```python
from build123d import *

# Parameters (mm, degrees)
SKETCH1_W           = 360
SKETCH1_H           = 210
BOSS_EXTRUDE1_DEPTH = 1
SKETCH2_R           = 5
SKETCH2_R_2         = 2.3
BOSS_EXTRUDE2_DEPTH = 5.7


with BuildPart() as part:
    # Sketch1 → Boss-Extrude1 (new body)
    with BuildSketch(Plane(origin=(0, 0, 0), x_dir=(1, 0, 0), z_dir=(0, 1, 0))):
        Rectangle(SKETCH1_W, SKETCH1_H)
        Polygon((28, -45.5), (0, -45.5), (0, 45.5), (-78.4, 45.5), (-78.4, -7.9), (-95, -7.9), (-95, 79.1), (-78.4, 79.1), (-78.4, 68.1), (28, 68.1), (28, 45.5), (66.5, 45.5), (66.5, -45.5), (66.5, -97), (28, -97), align=None, mode=Mode.SUBTRACT)
    extrude(amount=BOSS_EXTRUDE1_DEPTH)

    # Sketch2 → Boss-Extrude2 (add)
    with BuildSketch(Plane(origin=(0, 1, 0), x_dir=(1, 0, 0), z_dir=(0, 1, 0))):
        with Locations((-71.4, 75.1)):
            Circle(SKETCH2_R)
        with Locations((-71.4, 75.1)):
            Circle(SKETCH2_R_2, mode=Mode.SUBTRACT)
        with Locations((-71.4, 38.5)):
            Circle(SKETCH2_R)
        with Locations((-71.4, 38.5)):
            Circle(SKETCH2_R_2, mode=Mode.SUBTRACT)
        with Locations((-102, 75.1)):
            Circle(SKETCH2_R)
        with Locations((-102, 75.1)):
            Circle(SKETCH2_R_2, mode=Mode.SUBTRACT)
        with Locations((-7, 38.5)):
            Circle(SKETCH2_R)
        with Locations((-7, 38.5)):
            Circle(SKETCH2_R_2, mode=Mode.SUBTRACT)
        with Locations((35, 52.5)):
            Circle(SKETCH2_R)
        with Locations((35, 52.5)):
            Circle(SKETCH2_R_2, mode=Mode.SUBTRACT)
        with Locations((21, -52.5)):
            Circle(SKETCH2_R)
        with Locations((21, -52.5)):
            Circle(SKETCH2_R_2, mode=Mode.SUBTRACT)
        with Locations((-71.4, -0.9)):
            Circle(SKETCH2_R)
        with Locations((-71.4, -0.9)):
            Circle(SKETCH2_R_2, mode=Mode.SUBTRACT)
        with Locations((-102, -0.9)):
            Circle(SKETCH2_R)
        with Locations((-102, -0.9)):
            Circle(SKETCH2_R_2, mode=Mode.SUBTRACT)
        with Locations((73.5, -90)):
            Circle(SKETCH2_R)
        with Locations((73.5, -90)):
            Circle(SKETCH2_R_2, mode=Mode.SUBTRACT)
        with Locations((21, -90)):
            Circle(SKETCH2_R)
        with Locations((21, -90)):
            Circle(SKETCH2_R_2, mode=Mode.SUBTRACT)
    extrude(amount=BOSS_EXTRUDE2_DEPTH)


solid = part.part
```
Design review of the part built by this model. Coordinates are the model's own, in mm. A direction names the side the tool comes from. Coordinates: 2 decimals unless noted, no trailing zeros. Order: outer loops, then holes, each group sorted by start corner. A loop starts at its lowest first (then second) coordinate and runs counter-clockwise, first axis right, second up.
1) Take a section at B-B, the plane x = -86. Give the boundary of the cut face in (y, z), and give its area (3 significant figures).
2) For faces 1 (the cylindrical face through (78.119, 3.81, 91.915)), 2 (the flat face through (-70, 6.7, -73)), list the 3-axis set-ups (+Z, -Z, +X, -X, +Y, -Y) from which the entire face can be reached by the end or side of a thin tool; tool diameter is ignored.
3) Take a section at D-D, the plane x = 123. Give the boundary of the cut face in (y, z).
4) Take a section at C-C, the plane y = 3.75. State how many separate pieces and enclosed holes the cut face has, and give its area (3 significant figures).
5) Take a section at A-A, the plane z = 80. Give the boundary of the cut face in (x, y), and give its area (4 significant figures).
6) Wall thickness on line 1 along X through (y, z) = (3.3, -75.1); line 2 along X through (y, z) = (5.2, 90); line 3 along X through (y, z) = (0.75, 75.5): over which ranges is each line inside the solid? List them lowest first.
7) Clearance check with flat-ended pins moving along their axes: pin 1 (1 mm diameter, centred on y = 3, z = 52.5, fed in from +X); pin 2 (3 mm diameter, centred on x = -33, z = 63.5, fed in from +Y); pin 3 (4 mm diameter, centred on x = -100, y = 4.5, fed in from +Z); pin 4 (4 mm diameter, centred on x = -91.5, z = -56.5, fed in from -Y). State where each tip first meets the part, or that it passes through.
8) Mouldability with a two-part tool opening along Z and no side actions: class faces 3 (the flat face through (-6, 6.7, -36)), 4 (the cylindrical face through (19.92, 3.81, 94.88)), 5 (the cylindrical face through (-4.312, 3.81, -42.716)), 6 (the cylindrical face through (20.349, 3.81, 47.543)) as +Z half, -Z half, draft (parallel to the pull), parting line (faces both ways), or undercut.
Returned:
1. outline: (0, -105) - (1, -105) - (1, -79.1) - (0, -79.1) - close; (0, 7.9) - (1, 7.9) - (1, 105) - (0, 105) - close
1. area: 123 mm2
2. face 1: +Y
2. face 2: +Z, -Z, +X, -X, +Y
3. outline: (0, -105) - (1, -105) - (1, 105) - (0, 105) - close
4. separate pieces: 10
4. enclosed holes: 10
4. area: 619 mm2
5. outline: (-180, 0) - (28, 0) - (28, 1) - (-180, 1) - close; (66.5, 0) - (180, 0) - (180, 1) - (66.5, 1) - close
5. area: 321.5 mm2
6. line 1: x = -107 to -104.3, -99.7 to -97, -76.4 to -73.7, -69.1 to -66.4
6. line 2: x = 16 to 18.7, 23.3 to 26, 68.5 to 71.2, 75.8 to 78.5
6. line 3: x = -180 to 28, 66.5 to 180
7. pin 1: stops at x = 26
7. pin 2: stops at y = 1
7. pin 3: stops at z = 5.9
7. pin 4: passes through
8. face 3: draft
8. face 4: undercut
8. face 5: parting line
8. face 6: undercut
